Autodesk Inventor part; units mm, degrees
ref_plane "YZ Plane" through (0, 0, 0) normal (1, 0, 0) x (0, 1, 0)
ref_plane "XZ Plane" through (0, 0, 0) normal (0, 1, 0) x (-1, 0, 0)
ref_plane "XY Plane" through (0, 0, 0) normal (0, 0, 1) x (1, 0, 0)
sketch "Sketch_58" plane through (0, 0, 0) normal (0, 0, 1) x (1, 0, 0)
  line L0 (50, 0) -> (-50, 0)
  line L1 (0, 13.5683) -> (0, 12.7)
  arc A0 (0, 12.7) -> (0.2, 12.5) centre (0.2, 12.7) ccw
  line L2 (0.2, 12.5) -> (3.8, 12.5)
  arc A1 (3.8, 12.5) -> (4, 12.7) centre (3.8, 12.7) ccw
  line L3 (4, 12.7) -> (4, 13.5683)
  arc A2 (4, 13.5683) -> (3.9333, 13.635) centre (3.9333, 13.5683) ccw
  line L4 (3.9333, 13.635) -> (2.5022, 13.635)
  arc A3 (1.4978, 13.635) -> (2.5022, 13.635) centre (2, 14.25) ccw
  line L5 (1.4978, 13.635) -> (0.0667, 13.635)
  arc A4 (0.0667, 13.635) -> (0, 13.5683) centre (0.0667, 13.5683) ccw
revolve "Revolution1" add sketch "Sketch_58" angle 360 about axis through (50, 0, 0) along (1, 0, 0)
sketch "Sketch_60" plane through (0, 0, 0) normal (0, 0, 1) x (1, 0, 0)
  line L0 (50, 0) -> (-50, 0)
  line L1 (0.18, 15.145) -> (0.21, 14.7675)
  line L2 (0.21, 14.7675) -> (0.18, 14.39)
  line L3 (0.18, 14.39) -> (0.18, 13.635)
  line L4 (0.18, 13.635) -> (0.24, 13.635)
  line L5 (0.24, 13.635) -> (0.3, 14.39)
  line L6 (0.3, 14.39) -> (0.3, 14.7675)
  line L7 (0.3, 14.7675) -> (0.24, 15.145)
  line L8 (0.24, 15.145) -> (0.18, 15.145)
revolve "Revolution2" add sketch "Sketch_60" angle 360 about axis through (50, 0, 0) along (1, 0, 0)
sketch "Sketch_61" plane through (0, 0, 0) normal (0, 0, 1) x (1, 0, 0)
  line L0 (50, 0) -> (-50, 0)
  line L1 (3.7, 14.39) -> (3.76, 13.635)
  line L2 (3.76, 13.635) -> (3.82, 13.635)
  line L3 (3.82, 13.635) -> (3.82, 14.39)
  line L4 (3.82, 14.39) -> (3.79, 14.7675)
  line L5 (3.79, 14.7675) -> (3.82, 15.145)
  line L6 (3.82, 15.145) -> (3.76, 15.145)
  line L7 (3.76, 15.145) -> (3.7, 14.7675)
  line L8 (3.7, 14.7675) -> (3.7, 14.39)
revolve "Revolution3" add sketch "Sketch_61" angle 360 about axis through (50, 0, 0) along (1, 0, 0)
properties part number "W 61705-2RZ_PART1" material "Stainless Steel"
Model file for the job. Use its own axes, mm. A direction names the side the tool comes from. Coordinates: 2 decimals unless noted, no trailing zeros. Order: outer loops, then holes, each group sorted by start corner. A loop starts at its lowest first (then second) coordinate and runs counter-clockwise, first axis right, second up. Notation, with made-up numbers: M 30,13 L 47,13 A12 cw 47,28 Z; hole C -39,86 d9. An arc over 180 degrees is marked long. Answer as CSV lines item,"result".
(1) Band-saw the part on A-A, the plane x = 3. List the corners of the cut face in (y, z) (3 decimals).
Geometry says:
outline,"C 0,0 d27.27; hole C 0,0 d25"
(2) Wall check: line 1 along Z through (x, y) = (1.35, 0) (3 decimals); line 2 along Y through (x, z) = (2.25, -2.5); line 3 along Z through (x, y) = (2.3, -8). Give the ranges that are in metal, low to high.
Geometry says:
line 1,"z = -13.635 to -12.5, 12.5 to 13.635"
line 2,"y = -13.26 to -12.25, 12.25 to 13.26"
line 3,"z = -10.89 to -9.6, 9.6 to 10.89"
(3) Flat gauge pins, fed straight in: pin 1 (9 mm diameter, centred on y = 6.5, z = -6.5, fed in from -X); pin 2 (3 mm diameter, centred on y = -5, z = 9, fed in from -X); pin 3 (1.5 mm diameter, centred on x = 1.5, y = 12, fed in from +Z). Where does each tip first touch, or does it go through?
Geometry says:
pin 1,"stops at x = 0"
pin 2,"passes through"
pin 3,"stops at z = 7.7"
(4) 3-axis set-ups, long thin cutter, end or side, ignore diameter. For faces 3 (the cylindrical face through (3.12, -10.82, 8.3)), 4 (the flat face through (4, 5, -12)): which of +Z, -Z, +X, -X, +Y, -Y reach the whole face in a straight line?
Geometry says:
face 3,"none"
face 4,"+Z, -Z, +X, +Y, -Y"
(5) Pull direction Z, two halves, no side cores. Call faces 1 (the flat face through (0, 5, -12)), 2 (the cylindrical face through (2.025, 11.923, 3.755)): +Z half, -Z half, draft (parallel to the pull), parting line (faces both ways), or undercut.
Geometry says:
face 1,"draft"
face 2,"undercut"
